Verification items for the finished model (mm, model axes). A direction names the side the tool comes from. Give positions to 0.01 mm unless a question says otherwise; leave off trailing zeros. Write each loop counter-clockwise with the first axis right and the second up, starting at its lowest first coordinate (ties: lowest second). Pieces come first, ordered by that corner, then holes. Notation, with made-up numbers: M -32,67.25 L -17,67.25 A5 ccw -17,71.25 Z; hole C 23,-34 d3. An arc over 180 degrees is marked long. Answer as a JSON object with one key per item and string values.
```python
from build123d import *

# Parameters (mm, degrees)
BOSS_EXTRUDE2_DEPTH = 5
CUT_EXTRUDE1_DEPTH  = 2
SKETCH3_R           = 0.75
CUT_EXTRUDE2_DEPTH  = 33.350678515


with BuildPart() as part:
    # Sketch1 → Boss-Extrude2 (new body)
    with BuildSketch(Plane.XY):
        with BuildLine():
            Line((-23.25, 4.75), (-23.25, -4.75))
            Line((-23.25, -4.75), (-11.691342951, -4.75))
            ThreePointArc((-11.691342951, -4.75), (-9.949887623, -5.766468943), (-9.978567551, -7.78266666))
            Line((-9.978567551, -7.78266666), (-15.863620668, -17.543584287))
            Line((-15.863620668, -17.543584287), (-7.636379332, -22.293584287))
            Line((-7.636379332, -22.293584287), (-1.857050808, -12.283493649))
            ThreePointArc((-1.857050808, -12.283493649), (-0.106035217, -11.283583567), (1.625703261, -12.316519972))
            Line((1.625703261, -12.316519972), (7.136379332, -22.293584287))
            Line((7.136379332, -22.293584287), (15.363620668, -17.543584287))
            Line((15.363620668, -17.543584287), (9.584292144, -7.533493649))
            ThreePointArc((9.584292144, -7.533493649), (9.593852406, -5.517114624), (11.354270812, -4.533853312))
            Line((11.354270812, -4.533853312), (22.75, -4.75))
            Line((22.75, -4.75), (22.75, 4.75))
            Line((22.75, 4.75), (11.354270812, 4.533853312))
            ThreePointArc((11.354270812, 4.533853312), (9.593852406, 5.517114624), (9.584292144, 7.533493649))
            Line((9.584292144, 7.533493649), (15.363620668, 17.543584287))
            Line((15.363620668, 17.543584287), (7.136379332, 22.293584287))
            Line((7.136379332, 22.293584287), (1.625703261, 12.316519972))
            ThreePointArc((1.625703261, 12.316519972), (-0.106035217, 11.283583567), (-1.857050808, 12.283493649))
            Line((-1.857050808, 12.283493649), (-7.636379332, 22.293584287))
            Line((-7.636379332, 22.293584287), (-15.863620668, 17.543584287))
            Line((-15.863620668, 17.543584287), (-9.978567551, 7.78266666))
            ThreePointArc((-9.978567551, 7.78266666), (-9.949887623, 5.766468943), (-11.691342951, 4.75))
            Line((-11.691342951, 4.75), (-23.25, 4.75))
        make_face()
    extrude(amount=BOSS_EXTRUDE2_DEPTH)

    # Sketch2 → Cut-Extrude1 (cut)
    with BuildSketch(Plane(origin=(0, 0, 0), x_dir=(-1, 0, 0), z_dir=(0, 0, -1))):
        with BuildLine():
            Line((0.780612245, 4.177696078), (12.617346939, 1.965974625))
            ThreePointArc((12.617346939, 1.965974625), (14.25, 0), (12.617346939, -1.965974625))
            Line((12.617346939, -1.965974625), (0.780612245, -4.177696078))
            ThreePointArc((0.780612245, -4.177696078), (0, -4.25), (-0.780612245, -4.177696078))
            Line((-0.780612245, -4.177696078), (-12.617346939, -1.965974625))
            ThreePointArc((-12.617346939, -1.965974625), (-14.25, 0), (-12.617346939, 1.965974625))
            Line((-12.617346939, 1.965974625), (-0.780612245, 4.177696078))
            ThreePointArc((-0.780612245, 4.177696078), (0, 4.25), (0.780612245, 4.177696078))
        make_face()
    extrude(amount=-CUT_EXTRUDE1_DEPTH, mode=Mode.SUBTRACT)

    # Sketch3 → Cut-Extrude2 (cut, through all)
    with BuildSketch(Plane(origin=(0, 0, 2), x_dir=(-1, 0, 0), z_dir=(0, 0, -1))):
        with Locations((-6.5, 0)):
            Circle(SKETCH3_R)
        with Locations((-12.5, 0)):
            Circle(SKETCH3_R)
        with Locations(Location((6.5, 0, 0), (0, 0, 180))):
            Circle(SKETCH3_R)
        with Locations(Location((12.5, 0, 0), (0, 0, 180))):
            Circle(SKETCH3_R)
    extrude(amount=-CUT_EXTRUDE2_DEPTH, mode=Mode.SUBTRACT)


solid = part.part
```
1) Section check D-D on x = -2.5. Record the boundary of the cut face in (y, z).
Completed:
{"outline": "M -13.4,0 L -3.86,0 L -3.86,2 L 3.86,2 L 3.86,0 L 13.4,0 L 13.4,5 L -13.4,5 Z"}
2) Section check C-C on x = 6.5. Record the boundary of the cut face in (y, z), and give its area (3 significant figures).
Completed:
{"outline": "M -21.14,0 L -3.11,0 L -3.11,2 L -0.75,2 L -0.75,5 L -21.14,5 Z; M 0.75,2 L 3.11,2 L 3.11,0 L 21.14,0 L 21.14,5 L 0.75,5 Z", "area": "194 mm2"}
3) Section check A-A on y = 0. Record the boundary of the cut face in (x, z).
Completed:
{"outline": "M -23.25,0 L -14.25,0 L -14.25,2 L -13.25,2 L -13.25,5 L -23.25,5 Z; M -11.75,2 L -7.25,2 L -7.25,5 L -11.75,5 Z; M -5.75,2 L 5.75,2 L 5.75,5 L -5.75,5 Z; M 7.25,2 L 11.75,2 L 11.75,5 L 7.25,5 Z; M 13.25,2 L 14.25,2 L 14.25,0 L 22.75,0 L 22.75,5 L 13.25,5 Z"}
4) Thickness scan on L1, parallel to Y at x = 9.5, z = 0.4; L2, parallel to Y at x = -12.5, z = 4.3; L3, parallel to Y at x = -10, z = 3.1. Record the ranges inside material, lowest first.
Completed:
{"L1": "y = -20.93 to -7.37, -5.7 to -2.55, 2.55 to 5.7, 7.37 to 20.93", "L2": "y = -19.49 to -11.96, -4.75 to -0.75, 0.75 to 4.75, 11.96 to 19.49", "L3": "y = -20.93 to -7.82, -5.68 to 5.68, 7.82 to 20.93"}
5) Access from +Z, -Z, +X, -X, +Y, -Y to the whole of each face (thin tool, end or side, straight path). Record for faces 4 (the face through (12.434, 12.468, 2.465)), 5 (the face through (-4.706, 17.218, 2.465)), 6 (the face through (4.342, -17.235, 2.465)), 7 (the face through (-12.96, 12.73, 2.46)).
Completed:
{"face 4": "+Z, -Z, +X", "face 5": "+Z, -Z, +Y", "face 6": "+Z, -Z, -Y", "face 7": "+Z, -Z, -X"}
6) Release check for a two-part mould opening along X. For faces 1 (the face through (12.514, -12.609, 2.465)), 2 (the face through (-11.808, -19.885, 2.465)), 3 (the face through (7.25, 0.03, 3.48)) record: pulls with the +X half, pulls with the -X half, needs draft (parallel to the pull), parting line crosses it, or undercut.
Completed:
{"face 1": "pulls with the +X half", "face 2": "pulls with the -X half", "face 3": "undercut"}
7) Go/stop test with flat-tipped pins: pin 1 (7 mm diameter, centred on x = -5.5, y = 2, fed in from -Z); pin 2 (1.5 mm diameter, centred on x = -4, z = 1.5, fed in from -Y); pin 3 (1.5 mm diameter, centred on x = -16.5, z = 2, fed in from +Y); pin 4 (1.5 mm diameter, centred on x = -19, z = 1.5, fed in from -Y). Record where each tip stops, or that it passes through.
Completed:
{"pin 1": "stops at z = 0", "pin 2": "stops at y = -17.29", "pin 3": "stops at y = 17.61", "pin 4": "stops at y = -4.75"}
